Work out the finished part from the listing and answer in its coordinate system (mm). A direction names the side the tool comes from. Round coordinates to 2 decimals unless told otherwise and drop trailing zeros. One line per item, written item: value. Start each with the question number.
Q1. The mould has two halves that part along X. Classify faces 1 (the cylindrical face through (90, -1, 0)), 2 (the flat face through (42, -1, 77.5)), 3 (the cylindrical face through (33.58, -1.23, 62.27)), 4 (the cylindrical face through (61, -1, -52)): released by +X, released by -X, zero draft, split by the parting line, or undercut.
Q2. Given pin 1 Ø5 at (x, z) = (58, -59.5) entering from +Y; pin 2 Ø1.5 at (x, y) = (52, -2) entering from +Z; pin 3 Ø1.2 at (x, y) = (48.5, -1) entering from +Z; pin 4 Ø0.5 at (y, z) = (-1, -36.5) entering from +X, each flat-ended and moving along its own axis, determine where each tip first touches the part or whether it passes through.
Q3. Consider probe 1 along Z at (x, y) = (76, -1.6); probe 2 along Z at (x, y) = (81, -1.5); probe 3 along X at (y, z) = (-1.15, 2). Determine where each line is inside the solid, lowest interval first.
Q4. Find section A-A (y = -0.5). Count the separate pieces of the cut face and the enclosed holes in it, and give its area (3 significant figures).
Q5. A tool of negligible diameter and unlimited length cuts with its end or side. For faces 5 (the flat face through (56.12, -1, -42)), 6 (the flat face through (59.609, -1.232, 18.835)), from which of +Z, -Z, +X, -X, +Y, -Y can it reach the whole face along a straight path? Write none if from no direction.
from build123d import *

# Parameters (mm, degrees)
F1_DEPTH = 2.5
F2_D     = 7
F3_D     = 7.5


with BuildPart() as f1:
    # F0 (on Front) → F1 (new body)
    with BuildSketch(Plane.XZ):
        with BuildLine():
            ThreePointArc((44.3332993401, -75.1925694933), (45.8953218526, -76.4841948767), (47.9012588134, -76.1936309943))
            ThreePointArc((47.9012588134, -76.1936309943), (89.9939017876, 1.0476836528), (46.1144673234, 77.2881355932))
            ThreePointArc((46.1144673234, 77.2881355932), (45.7445133706, 77.4460642084), (45.345892868, 77.5))
            Line((45.345892868, 77.5), (39.5109278697, 77.5))
            ThreePointArc((39.5109278697, 77.5), (38.8271106657, 77.3350633062), (38.2936755268, 76.8765253754))
            ThreePointArc((38.2936755268, 76.8765253754), (33.5821559497, 62.0508178423), (38.5502726955, 47.3091138504))
            ThreePointArc((38.5502726955, 47.3091138504), (38.7858981986, 47.059289436), (39.0721677836, 46.8696019548))
            ThreePointArc((39.0721677836, 46.8696019548), (40.2651851973, 46.3424047588), (41.5083731547, 45.9478022555))
            ThreePointArc((41.5083731547, 45.9478022555), (41.6750655835, 45.8941514704), (41.8343694623, 45.8214393893))
            ThreePointArc((41.8343694623, 45.8214393893), (49.9805703397, 39.922405473), (56.1769145362, 32))
            Line((56.1769145362, 32), (63.1382883672, 5.2967772755))
            ThreePointArc((63.1382883672, 5.2967772755), (59.0933773697, -17.6430529265), (44.1204665888, -35.4870731412))
            ThreePointArc((44.1204665888, -35.4870731412), (43.4927479121, -37.4870731412), (44.1204665888, -39.4870731412))
            Line((44.1204665888, -39.4870731412), (45.6204665888, -39.4870731412))
            ThreePointArc((45.6204665888, -39.4870731412), (47.3882335418, -38.7548400941), (48.1204665888, -36.9870731412))
            Line((48.1204665888, -36.9870731412), (48.1204665888, -35.9870731412))
            Line((48.1204665888, -35.9870731412), (52.1204665888, -35.9870731412))
            ThreePointArc((52.1204665888, -35.9870731412), (54.9488937136, -37.1586460164), (56.1204665888, -39.9870731412))
            Line((56.1204665888, -39.9870731412), (56.1204665888, -43.4870731412))
            ThreePointArc((56.1204665888, -43.4870731412), (55.3882335418, -45.2548400941), (53.6204665888, -45.9870731412))
            ThreePointArc((53.6204665888, -45.9870731412), (51.8526996359, -45.2548400941), (51.1204665888, -43.4870731412))
            Line((51.1204665888, -43.4870731412), (51.1204665888, -42.4870731412))
            Line((51.1204665888, -42.4870731412), (46.0075130443, -42.4870731412))
            ThreePointArc((46.0075130443, -42.4870731412), (45.830736349, -42.5602964459), (45.7575130443, -42.7370731412))
            Line((45.7575130443, -42.7370731412), (45.7575130443, -58.7020410289))
            ThreePointArc((45.7575130443, -58.7020410289), (45.647970263, -59.4339660836), (45.3289416157, -60.1017494533))
            ThreePointArc((45.3289416157, -60.1017494533), (42.7900537692, -67.5124966586), (44.3332993401, -75.1925694933))
        make_face()
        with BuildLine():
            ThreePointArc((58.1584893781, -61.6403112281), (55.5006372806, -62.6076902787), (54.53325823, -59.9498381811))
            Line((54.53325823, -59.9498381811), (57.9142043239, -52.6993758848))
            ThreePointArc((57.9142043239, -52.6993758848), (60.5720564215, -51.7319968342), (61.5394354721, -54.3898489318))
            Line((61.5394354721, -54.3898489318), (58.1584893781, -61.6403112281))
        make_face(mode=Mode.SUBTRACT)
        with BuildLine():
            ThreePointArc((78.683841012, -12.3700931974), (83.2746114855, -12.5933116091), (83.0513930738, -17.1840820826))
            Line((83.0513930738, -17.1840820826), (77.4967905139, -22.2235652309))
            ThreePointArc((77.4967905139, -22.2235652309), (72.9060200403, -22.0003468191), (73.1292384521, -17.4095763456))
            Line((73.1292384521, -17.4095763456), (78.683841012, -12.3700931974))
        make_face(mode=Mode.SUBTRACT)
    extrude(amount=F1_DEPTH)

    # F2 (through all)
    with Locations(Plane(origin=(0, 0, 0), x_dir=(1, 0, 0), z_dir=(0, 1, 0))):
        with Locations((64.3298934041, -52.5379906052), (78, -5)):
            Hole(F2_D / 2)

    # F3 (through all)
    with Locations(Plane(origin=(0, 0, 0), x_dir=(1, 0, 0), z_dir=(0, 1, 0))):
        with Locations((69.7928888027, 36.7811946296)):
            Hole(F3_D / 2)


solid = f1.part
The answers:
1. face 1: released by +X
1. face 2: zero draft
1. face 3: released by -X
1. face 4: undercut
2. pin 1: y = 0
2. pin 2: z = 73.98
2. pin 3: z = 76.19
2. pin 4: x = 82.38
3. probe 1: -48.21 to -22.99, -14.81 to 2.13, 7.87 to 48.21
3. probe 2: -39.23 to -19.05, -11.53 to 3.2, 6.8 to 39.23
3. probe 3: 63.31 to 76.2, 79.8 to 89.98
4. separate pieces: 1
4. enclosed holes: 5
4. area: 3,970 mm2
5. face 5: +Y, -Y
5. face 6: -X, +Y, -Y
